Could you check a few things on this drawing? It's one solid part, dimensions in mm from its lowest x, y, z. Coordinates: 2 decimals unless noted, no trailing zeros. Order: outer loops, then holes, each group sorted by start corner. A loop starts at its lowest first (then second) coordinate and runs counter-clockwise, first axis right, second up. Notation, with made-up numbers: (1, -38.75) - (39, -38.75) arc R24 ccw to (39, -0.75) - close; hole circle Ø1 at (-33, -8). An arc over 180 degrees is marked (long way). Return JSON: item names as keys, results as strings. Group by question number.
1) For pin 1 Ø1.5 at (x, y) = (18, 165.5) entering from -Z, with a flat end and sliding along its axis, tell me the tip position at first contact or that it passes through.
2) If I drill on line 1 along Y through (x, z) = (30.5, 6.35); line 2 along Y through (x, z) = (33, 6) (1 decimal), over which ranges is the centre line in solid material (lowest first)?
3) Imagine slicing it at A-A (z = 6.35). Write out the boundary of the cut face in (x, y), and give its area (4 significant figures).
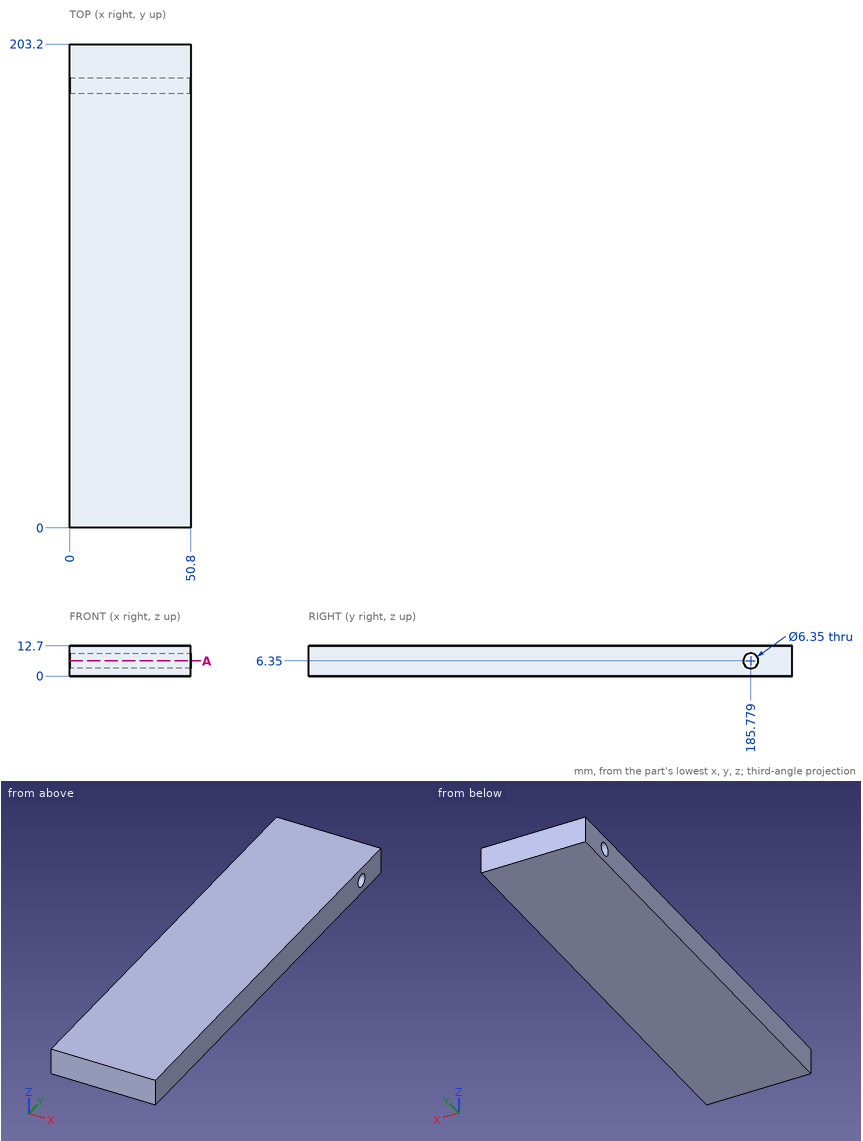
Calculated:
{
 "1": {"pin 1": "z = 0"},
 "2": {"line 1": "0 to 182.6, 188.95 to 203.2", "line 2": "0 to 182.6, 188.9 to 203.2"},
 "3": {"outline": "(0, 0) - (50.8, 0) - (50.8, 182.6) - (0, 182.6) - close; (0, 188.95) - (50.8, 188.95) - (50.8, 203.2) - (0, 203.2) - close", "area": "10,000 mm2"}
}
